Part print with two shaded views. Sizes in mm from the minimum x, y, z corner. Coordinates: 2 decimals unless noted, no trailing zeros. Loops run counter-clockwise (first coordinate to the right, second up) from the corner with the lowest first, then second, coordinate; pieces in that order, holes last. Notation, with made-up numbers: (12, 44) - (42, 44) arc R23 ccw to (42, 61) - close; hole circle Ø4 at (74.5, 78.25). An arc over 180 degrees is marked (long way). Answer as CSV lines item,"result".
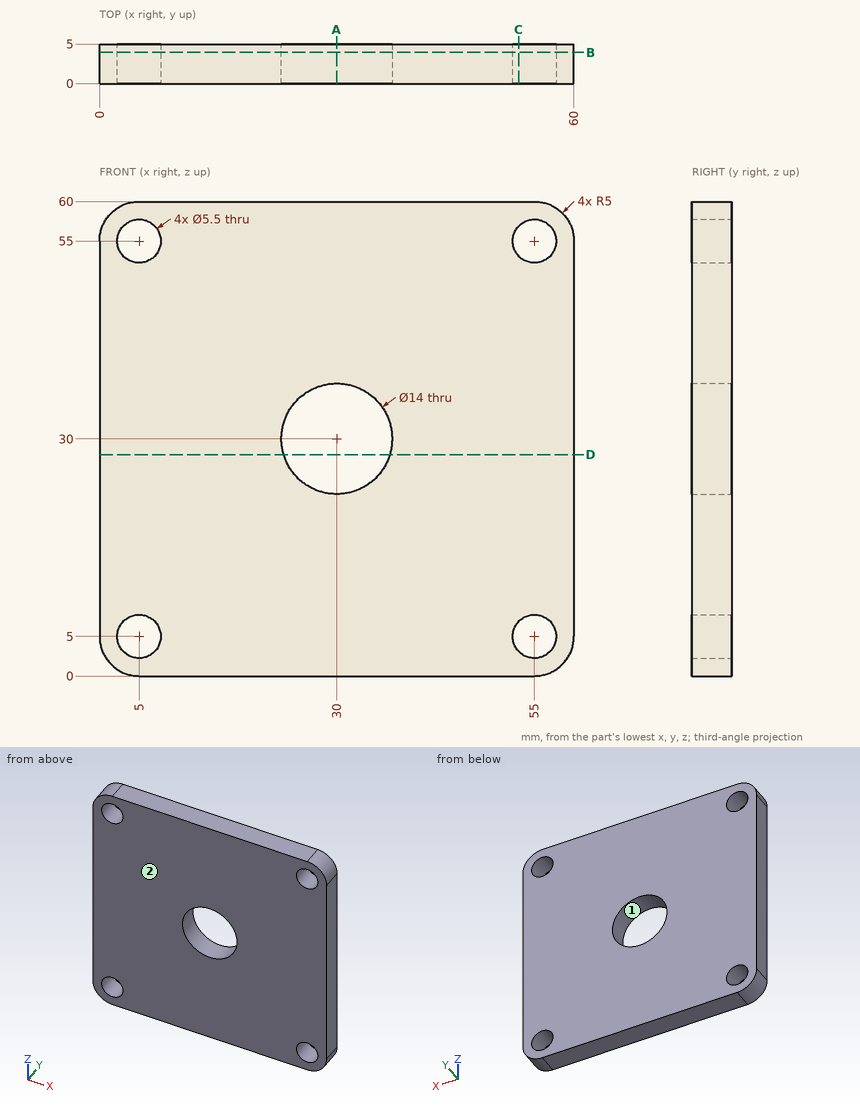
Q1. Wall check: L1, parallel to Z at x = 5, y = 2.35; L2, parallel to Z at x = 30, y = 2.1. Give the ranges that are in metal, low to high.
Results:
L1,"z = 0 to 2.25, 7.75 to 52.25, 57.75 to 60"
L2,"z = 0 to 23, 37 to 60"
Q2. Two-plate mould, pull along Z, no slides. Class the marked faces 1 and 2: released by +Z, released by -Z, zero draft, split by the parting line, or undercut.
Results:
face 1,"undercut"
face 2,"zero draft"
Q3. Saw through at B-B (y = 3.95). Give the cut face in (x, z), then the cut area to 3 significant figures.
Results:
outline,"(0, 5) arc R5 ccw to (5, 0) - (55, 0) arc R5 ccw to (60, 5) - (60, 55) arc R5 ccw to (55, 60) - (5, 60) arc R5 ccw to (0, 55) - close; hole circle Ø5.5 at (5, 5); hole circle Ø5.5 at (5, 55); hole circle Ø14 at (30, 30); hole circle Ø5.5 at (55, 5); hole circle Ø5.5 at (55, 55)"
area,"3,330 mm^2"
Q4. Flat gauge pin, fed straight in: pin 1 (7 mm diameter, centred on x = 55, z = 55, fed in from +Y). Where does the tip first touch, or does it go through?
Results:
pin 1,"stops at y = 5"
Q5. Saw through at D-D (z = 28). Give the cut face in (x, y), then the cut area to 3 significant figures.
Results:
outline,"(0, 0) - (23.29, 0) - (23.29, 5) - (0, 5) - close; (36.71, 0) - (60, 0) - (60, 5) - (36.71, 5) - close"
area,"233 mm^2"
Q6. Saw through at A-A (x = 30). Give the cut face in (y, z).
Results:
outline,"(0, 0) - (5, 0) - (5, 23) - (0, 23) - close; (0, 37) - (5, 37) - (5, 60) - (0, 60) - close"
Q7. Saw through at C-C (x = 53). Give the cut face in (y, z).
Results:
outline,"(0, 0) - (5, 0) - (5, 3.11) - (0, 3.11) - close; (0, 6.89) - (5, 6.89) - (5, 53.11) - (0, 53.11) - close; (0, 56.89) - (5, 56.89) - (5, 60) - (0, 60) - close"
